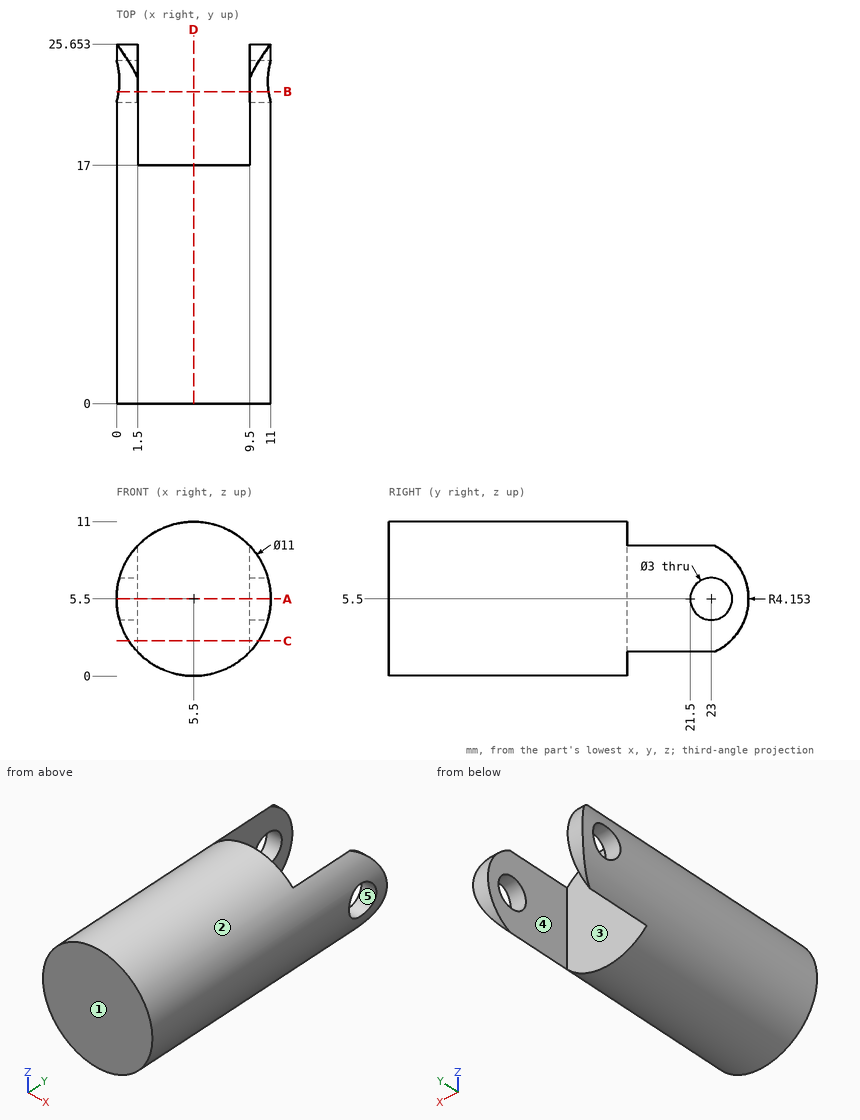
Study the drawing (mm; zero at the part's minimum x, y, z) and answer. A direction names the side the tool comes from. Coordinates: 2 decimals unless noted, no trailing zeros. Write each loop counter-clockwise with the first axis right and the second up, starting at its lowest first coordinate (ties: lowest second). Pieces come first, ordered by that corner, then holes.
Q1. Find the intervals of material crossed by line 1 (Y direction, x = 10.45, z = 5.5); line 2 (Y direction, x = 2.5, z = 1); line 3 (Z direction, x = 9.75, y = 23.25), in increasing order.
Q2. A cutting plane is placed at C-C, the plane z = 2.5. Give the vertices of the cut face in (x, y), then the cut area to 3 significant figures.
Q3. Determine the mould class of the marked faces 1, 2 and 3 for opening direction X: released by +X, released by -X, zero draft, split by the parting line, or undercut.
Q4. Which of the six approach directions +Z, -Z, +X, -X, +Y, -Y give full straight-line access (tool end or side, diameter ignored) to the marked faces 4 and 5?
Q5. A cutting plane is placed at B-B, the plane y = 22.25. Give the vertices of the cut face in (x, z) (1 decimal).
Q6. Each of these flat-tipped pins is pushed along its axis until it touches: pin 1 Ø6 at (x, z) = (3, 9) entering from +Y; pin 2 Ø1.8 at (y, z) = (23, 5.5) entering from +X; pin 3 Ø4 at (x, z) = (4.5, 6) entering from +Y; pin 4 Ø1.5 at (x, y) = (1.5, 19.5) entering from -Z (3 decimals). Where does it stop, or does it pass through?
Q7. A cutting plane is placed at D-D, the plane x = 5.5. Give the vertices of the cut face in (y, z).
Q8. A cutting plane is placed at A-A, the plane z = 5.5. Give the vertices of the cut face in (x, y), then the cut area to 3 significant figures.
Findings below:
1. line 1: y = 0 to 21.5, 24.5 to 25.65
1. line 2: y = 0 to 17
1. line 3: z = 2.01 to 4.02, 6.98 to 8.99
2. outline: (0.89, 0) - (10.11, 0) - (10.11, 24.37) - (9.5, 24.37) - (9.5, 17) - (1.5, 17) - (1.5, 24.37) - (0.89, 24.37) - close
2. area: 166 mm2
3. face 1: zero draft
3. face 2: split by the parting line
3. face 3: undercut
4. face 4: +Z, -Z, +Y
4. face 5: +X, -X
5. outline: (0.2, 4.2) arc R5.5 ccw to (1.5, 1.7) - (1.5, 4.2) - close; (0.2, 6.8) - (1.5, 6.8) - (1.5, 9.3) arc R5.5 ccw to start; (9.5, 1.7) arc R5.5 ccw to (10.8, 4.2) - (9.5, 4.2) - close; (9.5, 6.8) - (10.8, 6.8) arc R5.5 ccw to (9.5, 9.3) - close
6. pin 1: stops at y = 25.55
6. pin 2: passes through
6. pin 3: stops at y = 17
6. pin 4: stops at z = 1.725
7. outline: (0, 0) - (17, 0) - (17, 11) - (0, 11) - close
8. outline: (0, 0) - (11, 0) - (11, 21.5) - (9.5, 21.5) - (9.5, 17) - (1.5, 17) - (1.5, 21.5) - (0, 21.5) - close; (0, 24.5) - (1.5, 24.5) - (1.5, 25.65) - (0, 25.65) - close; (9.5, 24.5) - (11, 24.5) - (11, 25.65) - (9.5, 25.65) - close
8. area: 204 mm2
